```python
from build123d import *

# Parameters (mm, degrees)
SKETCH_1_R               = 25
EXTRUDE_1_DEPTH          = 30
SKETCH_2_R               = 25
EXTRUDE_2_DEPTH          = 250
SKETCH_3_W               = 40
SKETCH_3_H               = 10
EXTRUDE_4_DEPTH          = 40
CUT_EXTRUDE_1_DEPTH      = 323.877685819
CUT_EXTRUDE_1_DEPTH_BACK = 323.877685819
CUT_EXTRUDE_2_DEPTH      = 323.877685819
CUT_EXTRUDE_2_DEPTH_BACK = 323.877685819
SKETCH_7_R               = 10
SKETCH_8_R               = 25
CUT_EXTRUDE_3_DEPTH      = 180
SKETCH_9_R               = 15
CUT_EXTRUDE_4_DEPTH      = 30
FILLET_1_R               = 2.5


with BuildPart() as part:
    # 스케치1 → 보스-돌출1 (new body)
    with BuildSketch(Plane.XY):
        Circle(SKETCH_1_R)
    extrude(amount=-EXTRUDE_1_DEPTH)

    # 스케치2 → 보스-돌출2 (add)
    with BuildSketch(Plane(origin=(0, 0, -30), x_dir=(-1, 0, 0), z_dir=(0, 0, -1))):
        with Locations(Location((0, 0, 0), (0, 0, 180))):
            Circle(SKETCH_2_R)
    extrude(amount=EXTRUDE_2_DEPTH)

    # 스케치3 → 보스-돌출4 (add)
    with BuildSketch(Plane(origin=(0, 0, -280), x_dir=(-1, 0, 0), z_dir=(0, 0, -1))):
        with Locations((0, -5)):
            Rectangle(SKETCH_3_W, SKETCH_3_H)
        with Locations((0, 5)):
            Rectangle(SKETCH_3_W, SKETCH_3_H)
    extrude(amount=EXTRUDE_4_DEPTH)

    # 스케치6 → 컷-돌출1 (cut, two sides: drawn at the far end of the back side and taken through both)
    with BuildSketch(Plane(origin=(0, 10, 0), x_dir=(1, 0, 0), z_dir=(0, 1, 0)).offset(-CUT_EXTRUDE_1_DEPTH_BACK)):
        with BuildLine():
            ThreePointArc((-20, 300), (-14.142135624, 314.142135624), (0, 320))
            Line((0, 320), (-20, 320))
            Line((-20, 320), (-20, 300))
        make_face()
        with BuildLine():
            Line((20, 320), (0, 320))
            ThreePointArc((0, 320), (14.142135624, 314.142135624), (20, 300))
            Line((20, 300), (20, 320))
        make_face()
    extrude(amount=CUT_EXTRUDE_1_DEPTH + CUT_EXTRUDE_1_DEPTH_BACK, mode=Mode.SUBTRACT)

    # 스케치7 → 컷-돌출2 (cut, two sides: drawn at the far end of the back side and taken through both)
    with BuildSketch(Plane(origin=(0, 10, 0), x_dir=(1, 0, 0), z_dir=(0, 1, 0)).offset(-CUT_EXTRUDE_2_DEPTH_BACK)):
        with Locations(Location((0, 300, 0), (0, 0, 270))):
            Circle(SKETCH_7_R)
    extrude(amount=CUT_EXTRUDE_2_DEPTH + CUT_EXTRUDE_2_DEPTH_BACK, mode=Mode.SUBTRACT)

    # 스케치8 → 컷-돌출3 (cut)
    with BuildSketch(Plane.XY):
        Circle(SKETCH_8_R)
    extrude(amount=-CUT_EXTRUDE_3_DEPTH, mode=Mode.SUBTRACT)

    # 스케치9 → 컷-돌출4 (cut)
    with BuildSketch(Plane.XY.offset(-180)):
        Circle(SKETCH_9_R)
    extrude(amount=-CUT_EXTRUDE_4_DEPTH, mode=Mode.SUBTRACT)

    # 필렛1
    fillet_1_edges = [part.edges().sort_by_distance(p)[0] for p in [
        (-15, 0, -180),
    ]]
    fillet(fillet_1_edges, radius=FILLET_1_R)


solid = part.part
```
Input: part model. Units: mm. Frame: model coordinates. A direction names the side the tool comes from. Round coordinates to 2 decimals unless told otherwise and drop trailing zeros. Loops run counter-clockwise (first coordinate to the right, second up) from the corner with the lowest first, then second, coordinate; pieces in that order, holes last. Notation, with made-up numbers: (-35, -7) - (24, -7) arc R24 cw to (24, 22) - close; hole circle Ø10 at (39, 29.25). An arc over 180 degrees is marked (long way). One line per item, written item: value. Start each with the question number.
(1) Ray query, line 1 (X direction, y = 5.5, z = -300); line 2 (Y direction, x = 0, z = -188.75); line 3 (Z direction, x = -1.5, y = -6). Return the intervals inside material, ascending. Write a range as [from, to].
(2) Section A-A, the plane y = 0. Return loops of the section in (x, z), plus the area to 3 significant figures.
(3) Section D-D, the plane x = -21.5. Return loops of the section in (y, z).
(4) Contact query for flat-ended pins moving along their axis: P1, Ø5, axis at x = -12.5, y = 4.5, coming from the +Z side; P2, Ø10, axis at y = 11.5, z = -301.5, coming from the +X side; P3, Ø12, axis at x = -7, z = -297.5, coming from the +Y side. Output: stop coordinate, or through.
(5) Section B-B, the plane z = -197.5. Return loops of the section in (x, y), plus the area to 3 significant figures.
(6) Access query for faces 1 (the flat face through (5, 10, -291)), 2 (the flat face through (20, 0, -290)), 3 (the flat face through (5, -10, -291)), 4 (the cylindrical face through (-14.985, 0.66, -196.058)), 5 (the cylindrical face through (0, 0, -310)). Directions: +Z, -Z, +X, -X, +Y, -Y. A direction counts if a zero-diameter tool reaches every point of the face in a straight line with its end or side. Return the directions, or none.
(7) Draft query along X for faces 6 (the flat face through (0, 11, -280)), 7 (the flat face through (-20, 0, -290)), 8 (the flat face through (0, 0, -210)). Return one class per face: +X half, -X half, draft (parallel to the pull), parting line (faces both ways), or undercut.
(8) Section C-C, the plane y = -20. Return loops of the section in (x, z), plus the area to 3 significant figures.
Results below:
1. line 1: [-20, -10], [10, 20]
1. line 2: [-25, -15], [15, 25]
1. line 3: [-319.94, -309.89], [-290.11, -210]
2. outline: (-25, -280) - (-20, -280) - (-20, -300) arc R20 ccw to (20, -300) - (20, -280) - (25, -280) - (25, -180) - (17.5, -180) arc R2.5 ccw to (15, -182.5) - (15, -210) - (-15, -210) - (-15, -182.5) arc R2.5 ccw to (-17.5, -180) - (-25, -180) - close; hole circle Ø20 at (0, -300)
2. area: 5,210 mm^2
3. outline: (-12.76, -280) - (12.76, -280) - (12.76, -180) - (-12.76, -180) - close
4. P1: z = -180.68
4. P2: x = 20
4. P3: y = 10
5. outline: circle Ø50 at (0, 0); hole circle Ø30 at (0, 0)
5. area: 1,260 mm^2
6. face 1: -Z, +X, -X, +Y
6. face 2: -Z, +X, +Y, -Y
6. face 3: -Z, +X, -X, -Y
6. face 4: +Z
6. face 5: +Y, -Y
7. face 6: draft
7. face 7: -X half
7. face 8: undercut
8. outline: (-15, -280) - (15, -280) - (15, -180) - (-15, -180) - close
8. area: 3,000 mm^2
